```python
from build123d import *

# Parameters (mm, degrees)
SKETCH1_R           = 20
BOSS_EXTRUDE1_DEPTH = 3
CUT_EXTRUDE1_DEPTH  = 4
CIRPATTERN1_COUNT   = 30
SKETCH7_R           = 1.275
CUT_EXTRUDE6_DEPTH  = 4


with BuildPart() as part:
    # Sketch1 → Boss-Extrude1 (new body)
    with BuildSketch(Plane(origin=(0, 0, 0), x_dir=(1, 0, 0), z_dir=(0, 1, 0))):
        Circle(SKETCH1_R)
    extrude(amount=BOSS_EXTRUDE1_DEPTH)

    # Sketch2 → Cut-Extrude1 (cut, through all)
    with BuildSketch(Plane(origin=(0, 3, 0), x_dir=(1, 0, 0), z_dir=(0, 1, 0))):
        with BuildLine():
            ThreePointArc((-0.506578607, 17.180033014), (0, 17.1875), (0.506578607, 17.180033014))
            ThreePointArc((0.506578607, 17.180033014), (0.934108373, 18.613100259), (1.637465265, 19.932854976))
            ThreePointArc((1.637465265, 19.932854976), (0, 20), (-1.637465265, 19.932854976))
            ThreePointArc((-1.637465265, 19.932854976), (-0.934108373, 18.613100259), (-0.506578607, 17.180033014))
        make_face()
    cut_extrude1 = extrude(amount=-CUT_EXTRUDE1_DEPTH, mode=Mode.SUBTRACT)

    # CirPattern1: Cut-Extrude1 ×30 about axis
    cirpattern1_axis = Axis((0, 0, 0), (0, 1, 0))
    for i in range(1, CIRPATTERN1_COUNT):
        add(cut_extrude1.rotate(cirpattern1_axis, i * 360 / CIRPATTERN1_COUNT), mode=Mode.SUBTRACT)

    # Sketch7 → Cut-Extrude6 (cut, through all)
    with BuildSketch(Plane(origin=(0, 3, 0), x_dir=(1, 0, 0), z_dir=(0, 1, 0))):
        Circle(SKETCH7_R)
    extrude(amount=-CUT_EXTRUDE6_DEPTH, mode=Mode.SUBTRACT)


solid = part.part
```
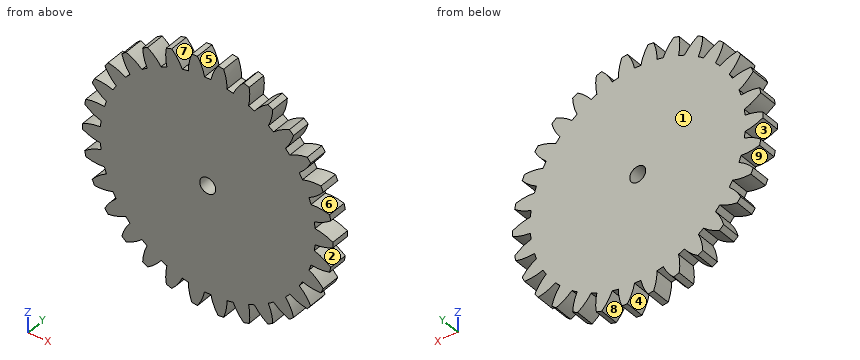
Part model, mm, in its own coordinate system. Face numbers are marked on the shaded views. A direction names the side the tool comes from. Coordinates: 2 decimals unless noted, no trailing zeros. Order: outer loops, then holes, each group sorted by start corner. A loop starts at its lowest first (then second) coordinate and runs counter-clockwise, first axis right, second up. Notation, with made-up numbers: (51.5, 7) -> (103.5, 7) arc R27 cw to (103.5, 24) -> close; hole circle Ø4 at (32, -15.5). An arc over 180 degrees is marked (long way). Put each result on its own line as item: value. Start each with the question number.
(1) Mould opens along Z. For the marked faces 6, 7, 8 and 9 say: pulls with the +Z half, pulls with the -Z half, needs draft (parallel to the pull), parting line crosses it, or undercut.
(2) Band-saw the part on C-C (z = -7). Give the cut face in (x, y), then the cut area to 3 significant figures.
(3) Probe line 1 along Z through (x, y) = (0, 2.2) (1 decimal); line 2 along Z through (x, y) = (12.5, 1.8); line 3 along Z through (x, y) = (17.5, 1.45). List the from-to ranges inside material, lowest first. Write a range as [from, to].
(4) Which spindle directions (+Z, -Z, +X, -X, +Y, -Y) get a long thin tool onto all of the face, cutting with end or side? Do the marked faces 1, 2, 3, 4 and 5. Say none if no direction does.
(5) Band-saw the part on B-B (z = 0). Give the cut face in (x, y) (3 decimals), then the cut area to 3 significant figures.
(6) Band-saw the part on A-A (x = 0). Give the cut face in (y, z) (1 decimal), then the cut area to 3 significant figures.
Determined:
1. face 6: undercut
1. face 7: pulls with the +Z half
1. face 8: pulls with the -Z half
1. face 9: undercut
2. outline: (-17.81, 0) -> (17.81, 0) -> (17.81, 3) -> (-17.81, 3) -> close
2. area: 107 mm²
3. line 1: z = [-17.2, -1.3], [1.3, 17.2]
3. line 2: z = [-14.94, -11.97], [-11.8, 11.8], [11.97, 14.94]
3. line 3: z = [-8.56, -6.71], [-4.88, -2.46], [-1.25, 1.25], [2.46, 4.88], [6.71, 8.56]
4. face 1: +Z, -Z, +X, -X, +Y
4. face 2: +X, +Y, -Y
4. face 3: -X, +Y, -Y
4. face 4: -Z, +Y, -Y
4. face 5: +Z, +Y, -Y
5. outline: (-20, 0) -> (-1.275, 0) -> (-1.275, 3) -> (-20, 3) -> close; (1.275, 0) -> (20, 0) -> (20, 3) -> (1.275, 3) -> close
5. area: 112 mm²
6. outline: (0, -17.2) -> (3, -17.2) -> (3, -1.3) -> (0, -1.3) -> close; (0, 1.3) -> (3, 1.3) -> (3, 17.2) -> (0, 17.2) -> close
6. area: 95.5 mm²
